Model file for the job. Use its own axes, mm. Coordinates: 2 decimals unless noted, no trailing zeros. Loops run counter-clockwise (first coordinate to the right, second up) from the corner with the lowest first, then second, coordinate; pieces in that order, holes last. Notation, with made-up numbers: (29, 58) -> (65, 58) arc R16 cw to (65, 87) -> close; hole circle Ø3 at (-23, 62.5). An arc over 180 degrees is marked (long way). Use one line per item in the form item = value.
```python
from build123d import *

# Parameters (mm, degrees)
BOSS_EXTRUDE1_DEPTH = 3.175
SKETCH1_4_R         = 3.5
CUT_EXTRUDE1_DEPTH  = 439.905857431
FILLET1_R           = 48
CUT_EXTRUDE3_DEPTH  = 10
CUT_EXTRUDE5_REACH  = 440.906
SKETCH11_R          = 5


with BuildPart() as part:
    # Sketch1 → Boss-Extrude1 (new body)
    with BuildSketch(Plane.XY):
        Polygon((-98.879411765, 3.850980392), (-31.879411765, -96.649019608), (366, -96.649019608), (403.120588235, -71.149019608), (428.120588235, 28.939617947), (-115.605170134, 28.939617947), align=None)
    extrude(amount=BOSS_EXTRUDE1_DEPTH)

    # Sketch1<4> → Cut-Extrude1 (cut, through all)
    with BuildSketch(Plane.XY):
        with Locations((3.120588235, -83.899019608)):
            Circle(SKETCH1_4_R)
        with Locations((67.120588235, -83.899019608)):
            Circle(SKETCH1_4_R)
        with Locations((131.120588235, -83.899019608)):
            Circle(SKETCH1_4_R)
        with Locations((195.120588235, -83.899019608)):
            Circle(SKETCH1_4_R)
        with Locations((259.120588235, -83.899019608)):
            Circle(SKETCH1_4_R)
        with Locations((323.120588235, -83.899019608)):
            Circle(SKETCH1_4_R)
    extrude(amount=CUT_EXTRUDE1_DEPTH, mode=Mode.SUBTRACT)

    # Fillet1
    fillet1_edges = [part.edges().sort_by_distance(p)[0] for p in [
        (-31.879411765, -96.649019608, 1.5875),
    ]]
    fillet(fillet1_edges, radius=FILLET1_R)

    # Sketch7 → Cut-Extrude3 (cut)
    with BuildSketch(Plane.XY.offset(3.175)):
        Polygon((403.120588235, -71.149019608), (340.005873473, -96.649019608), (366, -96.649019608), align=None)
    extrude(amount=-CUT_EXTRUDE3_DEPTH, mode=Mode.SUBTRACT)

    # Sketch11 → Cut-Extrude5 (cut, up to next)
    with BuildSketch(Plane(origin=(0, 0, 0), x_dir=(-1, 0, 0), z_dir=(0, 0, -1)), mode=Mode.PRIVATE) as cut_extrude5_sk1:
        with Locations((-397.678558137, -24.610405219)):
            Circle(SKETCH11_R)
    cut_extrude5_tool1 = extrude(cut_extrude5_sk1.sketch, amount=-CUT_EXTRUDE5_REACH, mode=Mode.PRIVATE) & part.part
    add(cut_extrude5_tool1.solids().sort_by_distance((397.678558, -24.610405, 0))[0], mode=Mode.SUBTRACT)


solid = part.part
```
Q1. Wall check: line 1 along X through (y, z) = (19.5, 0.85); line 2 along X through (y, z) = (6, 2.5); line 3 along Y through (x, z) = (354, 3). Give the ranges that are in metal, low to high.
Result:
line_1 = -109.31 to 425.76
line_2 = -100.31 to 422.39
line_3 = -91 to 28.94
Q2. Mould opens along Y. For faces 1 (the face through (152, -33, 3.175)), 2 (the face through (392.91, -23.11, 1.57)), 3 (the face through (415.446, -21.805, 1.565)) say: released by +Y, released by -Y, zero draft, split by the parting line, or undercut.
Result:
face_1 = zero draft
face_2 = undercut
face_3 = released by -Y
Q3. Band-saw the part on A-A, the plane z = 1.25. Write the cut outline in (x, y).
Result:
outline = (-115.61, 28.94) -> (-46.13, -75.27) arc R48 ccw to (-6.19, -96.65) -> (340.01, -96.65) -> (403.12, -71.15) -> (428.12, 28.94) -> close; hole circle Ø7 at (3.12, -83.9); hole circle Ø7 at (67.12, -83.9); hole circle Ø7 at (131.12, -83.9); hole circle Ø7 at (195.12, -83.9); hole circle Ø7 at (259.12, -83.9); hole circle Ø7 at (323.12, -83.9); hole circle Ø10 at (397.68, -24.61)
Q4. Band-saw the part on C-C, the plane y = -2. Write the cut outline in (x, z) (3 decimals).
Result:
outline = (-94.979, 0) -> (420.393, 0) -> (420.393, 3.175) -> (-94.979, 3.175) -> close
Q5. Pin check, flat tip, straight feed: pin 1 Ø10 at (x, y) = (282.5, 1) entering from -Z. Stop position of the tip, or through.
Result:
pin_1 = 0
Q6. Band-saw the part on B-B, the plane y = -43.5. Write the cut outline in (x, z) (3 decimals), and give its area (3 significant figures).
Result:
outline = (-67.312, 0) -> (410.027, 0) -> (410.027, 3.175) -> (-67.312, 3.175) -> close
area = 1,520 mm2
